Here's how the part is built. I have some questions about the finished solid (model axes, mm). Round coordinates to 2 decimals unless told otherwise and drop trailing zeros. Loops run counter-clockwise (first coordinate to the right, second up) from the corner with the lowest first, then second, coordinate; pieces in that order, holes last. Notation, with made-up numbers: M 36,9.25 L 87,9.25 A27 ccw 87,31.25 Z; hole C 13,8 d8. An arc over 180 degrees is marked long. Write item = value, one per line. Start each with the question number.
from build123d import *

# Parameters (mm, degrees)
SKETCH_1_W      = 200
SKETCH_1_H      = 200
SKETCH_1_R      = 2.5
SKETCH_1_R_2    = 10
SKETCH_1_R_3    = 2.75
EXTRUDE_1_DEPTH = 3


with BuildPart() as part:
    # 草图1 → 凸台-拉伸1 (new body)
    with BuildSketch(Plane(origin=(0, 0, 0), x_dir=(1, 0, 0), z_dir=(0, 1, 0))):
        Rectangle(SKETCH_1_W, SKETCH_1_H)
        with Locations(Location((0, 60, 0), (0, 0, 270))):
            Circle(SKETCH_1_R, mode=Mode.SUBTRACT)
        with Locations(Location((50, 0, 0), (0, 0, 270))):
            Circle(SKETCH_1_R_2, mode=Mode.SUBTRACT)
        with Locations(Location((50, 16, 0), (0, 0, 270))):
            Circle(SKETCH_1_R_3, mode=Mode.SUBTRACT)
        with Locations(Location((50, -16, 0), (0, 0, 270))):
            Circle(SKETCH_1_R_3, mode=Mode.SUBTRACT)
        with Locations(Location((-50, -16, 0), (0, 0, 90))):
            Circle(SKETCH_1_R_3, mode=Mode.SUBTRACT)
        with Locations(Location((-50, 16, 0), (0, 0, 90))):
            Circle(SKETCH_1_R_3, mode=Mode.SUBTRACT)
        with Locations(Location((-50, 0, 0), (0, 0, 90))):
            Circle(SKETCH_1_R_2, mode=Mode.SUBTRACT)
    extrude(amount=EXTRUDE_1_DEPTH)


solid = part.part
Item 1: We'd pull the mould along Z, two halves only. Please class faces 1 (the flat face through (-1, 0, -1)), 2 (the cylindrical face through (-0.96, 1.48, -57.69)), 3 (the cylindrical face through (-52.727, 1.479, -15.642)): released by +Z, released by -Z, zero draft, split by the parting line, or undercut.
Item 2: I want a section at B-B, the plane x = 50. List the corners of the cut face in (y, z) for me, then the cut area to 3 significant figures.
Item 3: Please list where these lines run through material, in increasing order: line 1 (Z direction, x = -50, y = 0.65); line 2 (X direction, y = 1.2, z = 0.5); line 3 (X direction, y = 2.25, z = -16). Write a range as [from, to].
Item 4: I want a section at D-D, the plane x = 0. List the corners of the cut face in (y, z) for me, then the cut area to 3 significant figures.
Item 5: I want a section at C-C, the plane y = 1.5. List the corners of the cut face in (x, z) for me.
Item 6: Will this pin go through, and if not, where does the flat tip stop? pin 1 Ø4.5 at (x, z) = (-50, 16) entering from -Y.
Item 7: I want a section at A-A, the plane z = -16. List the corners of the cut face in (x, y) for me.
Worked out:
q1.face_1 = zero draft
q1.face_2 = undercut
q1.face_3 = undercut
q2.outline = M 0,-100 L 3,-100 L 3,-18.75 L 0,-18.75 Z; M 0,-13.25 L 3,-13.25 L 3,-10 L 0,-10 Z; M 0,10 L 3,10 L 3,13.25 L 0,13.25 Z; M 0,18.75 L 3,18.75 L 3,100 L 0,100 Z
q2.area = 507 mm2
q3.line_1 = [-100, -18.75], [-13.25, -10], [10, 13.25], [18.75, 100]
q3.line_2 = [-100, -59.99], [-40.01, 40.01], [59.99, 100]
q3.line_3 = [-100, -52.75], [-47.25, 47.25], [52.75, 100]
q4.outline = M 0,-100 L 3,-100 L 3,-62.5 L 0,-62.5 Z; M 0,-57.5 L 3,-57.5 L 3,100 L 0,100 Z
q4.area = 585 mm2
q5.outline = M -100,-100 L 100,-100 L 100,100 L -100,100 Z; hole C -50,0 d20; hole C -50,-16 d5.5; hole C -50,16 d5.5; hole C 0,-60 d5; hole C 50,0 d20; hole C 50,-16 d5.5; hole C 50,16 d5.5
q6.pin_1 = through
q7.outline = M -100,0 L -52.75,0 L -52.75,3 L -100,3 Z; M -47.25,0 L 47.25,0 L 47.25,3 L -47.25,3 Z; M 52.75,0 L 100,0 L 100,3 L 52.75,3 Z
